from build123d import *

# Parameters (mm, degrees)
SKETCH1_R               = 1.6
BOSS_EXTRUDE1_DEPTH     = 69
SKETCH2_W               = 21.169041722
SKETCH2_H               = 16.5
CUT_EXTRUDE1_DEPTH      = 61
TAP_DRILL_FOR_M3_TAP1_D = 2.5


with BuildPart() as part:
    # Sketch1 → Boss-Extrude1 (new body)
    with BuildSketch(Plane(origin=(0, 0, 0), x_dir=(0, 0, -1), z_dir=(1, 0, 0))):
        with BuildLine():
            Line((-5, 23.6), (-5, 12.823580437))
            ThreePointArc((-5, 12.823580437), (-5.734562511, 9.130685315), (-7.826419562, 5.999999999))
            Line((-7.826419562, 5.999999999), (-13.211861119, 0.614558441))
            ThreePointArc((-13.211861119, 0.614558441), (-13.28989931, 0.222233964), (-12.957302678, 0))
            Line((-12.957302678, 0), (-5.826419558, 0))
            Line((-5.826419558, 0), (-2.840921838, 2.98549772))
            Line((-2.840921838, 2.98549772), (-2.840921838, 4.98549772))
            ThreePointArc((-2.840921838, 4.98549772), (-2.694475228, 5.339051111), (-2.340921838, 5.48549772))
            Line((-2.340921838, 5.48549772), (-1.139311489, 5.48549772))
            ThreePointArc((-1.139311489, 5.48549772), (-0.785758099, 5.631944329), (-0.639311489, 5.98549772))
            Line((-0.639311489, 5.98549772), (-0.639311489, 9.98549772))
            ThreePointArc((-0.639311489, 9.98549772), (3.534390695, 16.231884461), (5, 23.6))
            ThreePointArc((5, 23.6), (0, 28.6), (-5, 23.6))
        make_face()
        with Locations((0, 23.6)):
            Circle(SKETCH1_R, mode=Mode.SUBTRACT)
    extrude(amount=BOSS_EXTRUDE1_DEPTH)

    # Sketch2 → Cut-Extrude1 (cut)
    with BuildSketch(Plane(origin=(4, 0, 0), x_dir=(0, 0, -1), z_dir=(1, 0, 0))):
        with Locations((-5.584520861, 20.35)):
            Rectangle(SKETCH2_W, SKETCH2_H)
    extrude(amount=CUT_EXTRUDE1_DEPTH, mode=Mode.SUBTRACT)

    # Tap Drill for M3 Tap1 (through all)
    with Locations(Plane(origin=(69, 0, 0), x_dir=(0, 0, -1), z_dir=(1, 0, 0))):
        with Locations((-1, 15.6)):
            Hole(TAP_DRILL_FOR_M3_TAP1_D / 2)


solid = part.part
Could you check a few things on this model? Use its own coordinates, in mm. A direction names the side the tool comes from. Give positions to 0.01 mm unless a question says otherwise; leave off trailing zeros. Loops run counter-clockwise (first coordinate to the right, second up) from the corner with the lowest first, then second, coordinate; pieces in that order, holes last. Notation, with made-up numbers: (-11, 38.25) -> (6, 38.25) arc R6 ccw to (6, 47.25) -> close; hole circle Ø1 at (88.25, 76). An arc over 180 degrees is marked (long way). Return JSON: item names as keys, results as strings.
Item 1: If we section it at A-A on z = -3.25: List the corners of the cut face in (x, y) for me.
Geometry results:
{"outline": "(0, 15.58) -> (4, 15.58) -> (4, 27.4) -> (0, 27.4) -> close; (65, 15.58) -> (69, 15.58) -> (69, 27.4) -> (65, 27.4) -> close"}
Item 2: If we section it at B-B on x = 51.5: List the corners of the cut face in (y, z) for me, plus the area to 3 significant figures.
Geometry results:
{"outline": "(0, 5.83) -> (2.99, 2.84) -> (4.99, 2.84) arc R0.5 cw to (5.49, 2.34) -> (5.49, 1.14) arc R0.5 ccw to (5.99, 0.64) -> (9.99, 0.64) arc R19.25 ccw to (12.1, -1.19) -> (12.1, 5.03) arc R9.65 cw to (6, 7.83) -> (0.61, 13.21) arc R0.36 ccw to (0, 12.96) -> close", "area": "79.0 mm²"}
Item 3: I need wall thicknesses on L1, parallel to X at y = 26.25, z = -3.5; L2, parallel to Y at x = 67.35, z = 1; L3, parallel to Z at x = 2.35, y = 23.6. Which ranges of each line are inside material? Lowest first, please. Write a range as from..to.
Geometry results:
{"L1": "x = 0..4, 65..69", "L2": "y = 5.51..14.35, 16.85..22.35, 24.85..28.5", "L3": "z = -5..-1.6, 1.6..5"}
Item 4: I'm going to push flat-ended pins straight in: pin 1 (4.5 mm diameter, centred on x = 27.5, y = 7.5, fed in from -Z); pin 2 (8 mm diameter, centred on y = 22, z = 0.5, fed in from -X); pin 3 (2 mm diameter, centred on y = 15.6, z = 1, fed in from -X); pin 4 (5 mm diameter, centred on x = 28.5, z = 2, fed in from +Y). Where does each tip first touch, or does it pass through?
Geometry results:
{"pin 1": "stops at z = 0.64", "pin 2": "stops at x = 0", "pin 3": "passes through", "pin 4": "stops at y = 12.1"}
Item 5: Which directions (+Z, -Z, +X, -X, +Y, -Y) give clear straight access to the entire face, cutting with the end or side of a thin tool? Please do faces 1 (the flat face through (4, 20, 0)), 2 (the cylindrical face through (1.972, 25.186, 0.208)), 3 (the flat face through (0, 14.5, 2.3)), 4 (the flat face through (67, 18, 5)), 5 (the flat face through (34, 4, 2.841)).
Geometry results:
{"face 1": "+Z, -Z, +Y", "face 2": "+X, -X", "face 3": "+Z, -Z, -X, +Y, -Y", "face 4": "+Z, +X, -X, +Y", "face 5": "-Z, +X, -X, -Y"}
Item 6: If we section it at C-C on y = 8.5: List the corners of the cut face in (x, z) for me.
Geometry results:
{"outline": "(0, 0.64) -> (69, 0.64) -> (69, 6.02) -> (0, 6.02) -> close"}
Item 7: We'd pull the mould along Z, two halves only. Please class faces 6 (the flat face through (2, 18, 5)), 7 (the cylindrical face through (66.972, 25.186, 0.208)), 8 (the flat face through (34, 5.485, 2)), 9 (the cylindrical face through (66.97, 16.84, 0.84)): +Z half, -Z half, draft (parallel to the pull), parting line (faces both ways), or undercut.
Geometry results:
{"face 6": "+Z half", "face 7": "undercut", "face 8": "draft", "face 9": "undercut"}
Item 8: If we section it at D-D on z = 8.5: List the corners of the cut face in (x, y) for me, plus the area to 3 significant figures.
Geometry results:
{"outline": "(0, 0) -> (69, 0) -> (69, 5.33) -> (0, 5.33) -> close", "area": "368 mm²"}
